Build history of the part. All positions in model axes, mm. Round coordinates to 2 decimals unless told otherwise and drop trailing zeros. Write each loop counter-clockwise with the first axis right and the second up, starting at its lowest first coordinate (ties: lowest second). Pieces come first, ordered by that corner, then holes. Notation, with made-up numbers: (14, 46) - (28, 46) arc R9 ccw to (28, 53) - close; hole circle Ø6 at (-9, 29.5). An arc over 180 degrees is marked (long way). Answer as a JSON object with one key per item and string values. Group by question number.
Item 1: Two-plate mould, pull along Z, no slides. Class faces 1 (the cylindrical face through (-31.156, 4.014, 32.365)), 2 (the flat face through (41, 33, 22)): +Z half, -Z half, draft (parallel to the pull), parting line (faces both ways), or undercut.
Item 2: Slice it at C-C, the plane y = 30. List the corners of the cut face in (x, z).
Item 3: Slice it at D-D, the plane x = 43.5. List the corners of the cut face in (y, z).
Item 4: Slice it at A-A, the plane z = 0. List the corners of the cut face in (x, y).
Item 5: Flat gauge pins, fed straight in: pin 1 (5 mm diameter, centred on x = 36, z = -23, fed in from +Y); pin 2 (2 mm diameter, centred on x = 20.5, y = 11.5, fed in from -Z); pin 3 (12 mm diameter, centred on y = 20.5, z = 27, fed in from -X). Where does each tip first touch, or does it go through?
Item 6: Probe line 1 (X direction, y = 2.3, z = 0); line 2 (Y direction, x = 3, z = 40); line 3 (Z direction, x = -8.5, y = 24). List the from-to ranges inside material, lowest first. Write a range as from..to.
Item 7: Slice it at B-B, the plane x = 0. List the corners of the cut face in (y, z), then the cut area to 3 significant figures.
from build123d import *

# Parameters (mm, degrees)
SKETCH1_R           = 50
BOSS_EXTRUDE1_DEPTH = 5
SKETCH2_R           = 2.5
BOSS_EXTRUDE2_DEPTH = 30
SKETCH3_R           = 50
BOSS_EXTRUDE3_DEPTH = 28
SKETCH4_R           = 39
CUT_EXTRUDE1_DEPTH  = 6
SKETCH5_R           = 3
CUT_EXTRUDE2_DEPTH  = 44
SKETCH6_R           = 50
SKETCH6_R_2         = 39
BOSS_EXTRUDE4_DEPTH = 3


with BuildPart() as part:
    # Sketch1 → Boss-Extrude1 (new body)
    with BuildSketch(Plane(origin=(0, 0, 0), x_dir=(1, 0, 0), z_dir=(0, 1, 0))):
        Circle(SKETCH1_R)
    extrude(amount=BOSS_EXTRUDE1_DEPTH)

    # Sketch2 → Boss-Extrude2 (add)
    with BuildSketch(Plane(origin=(0, 5, 0), x_dir=(1, 0, 0), z_dir=(0, 1, 0))):
        with Locations((43, 0)):
            Circle(SKETCH2_R)
        with Locations((36.173901912, -23.247555151)):
            Circle(SKETCH2_R)
        with Locations((17.862845559, -39.1141758)):
            Circle(SKETCH2_R)
        with Locations((-6.119538046, -42.562322001)):
            Circle(SKETCH2_R)
        with Locations((-28.15901156, -32.497231697)):
            Circle(SKETCH2_R)
        with Locations((-41.258197865, -12.114499944)):
            Circle(SKETCH2_R)
        with Locations((-41.258197865, 12.114499944)):
            Circle(SKETCH2_R)
        with Locations((-28.15901156, 32.497231697)):
            Circle(SKETCH2_R)
        with Locations((-6.119538046, 42.562322001)):
            Circle(SKETCH2_R)
        with Locations((17.862845559, 39.1141758)):
            Circle(SKETCH2_R)
        with Locations((36.173901912, 23.247555151)):
            Circle(SKETCH2_R)
    extrude(amount=BOSS_EXTRUDE2_DEPTH)

    # Sketch3 → Boss-Extrude3 (add)
    with BuildSketch(Plane(origin=(0, 5, 0), x_dir=(1, 0, 0), z_dir=(0, 1, 0))):
        Circle(SKETCH3_R)
        with BuildLine():
            ThreePointArc((45.918604651, -2.735278211), (47, 0), (45.918604651, 2.735278211))
            ThreePointArc((45.918604651, 2.735278211), (44.136676786, 12.959697615), (40.107991433, 22.524409497))
            ThreePointArc((40.107991433, 22.524409497), (39.538916043, 25.41011842), (37.150385338, 27.126534413))
            ThreePointArc((37.150385338, 27.126534413), (30.123593761, 34.76448042), (21.563374325, 40.632756339))
            ThreePointArc((21.563374325, 40.632756339), (19.524505611, 42.752703782), (16.587181171, 42.905307606))
            ThreePointArc((16.587181171, 42.905307606), (6.546482561, 45.531786327), (-3.827461772, 45.840490141))
            ThreePointArc((-3.827461772, 45.840490141), (-6.688797399, 46.521607768), (-9.242335817, 45.061948789))
            ThreePointArc((-9.242335817, 45.061948789), (-19.109090598, 41.843071786), (-28.0031058, 36.494192217))
            ThreePointArc((-28.0031058, 36.494192217), (-30.778454495, 35.520229995), (-32.137476487, 32.911739623))
            ThreePointArc((-32.137476487, 32.911739623), (-38.69766251, 24.869477603), (-43.287961597, 15.561246119))
            ThreePointArc((-43.287961597, 15.561246119), (-45.09616976, 13.241430172), (-44.829195445, 10.312285671))
            ThreePointArc((-44.829195445, 10.312285671), (-46, 0), (-44.829195445, -10.312285671))
            ThreePointArc((-44.829195445, -10.312285671), (-45.09616976, -13.241430172), (-43.287961597, -15.561246119))
            ThreePointArc((-43.287961597, -15.561246119), (-38.69766251, -24.869477603), (-32.137476487, -32.911739623))
            ThreePointArc((-32.137476487, -32.911739623), (-30.778454495, -35.520229995), (-28.0031058, -36.494192217))
            ThreePointArc((-28.0031058, -36.494192217), (-19.109090598, -41.843071786), (-9.242335817, -45.061948789))
            ThreePointArc((-9.242335817, -45.061948789), (-6.688797399, -46.521607768), (-3.827461772, -45.840490141))
            ThreePointArc((-3.827461772, -45.840490141), (6.546482561, -45.531786327), (16.587181171, -42.905307606))
            ThreePointArc((16.587181171, -42.905307606), (19.524505611, -42.752703782), (21.563374325, -40.632756339))
            ThreePointArc((21.563374325, -40.632756339), (30.123593761, -34.76448042), (37.150385338, -27.126534413))
            ThreePointArc((37.150385338, -27.126534413), (39.538916043, -25.41011842), (40.107991433, -22.524409497))
            ThreePointArc((40.107991433, -22.524409497), (44.136676786, -12.959697615), (45.918604651, -2.735278211))
        make_face(mode=Mode.SUBTRACT)
    extrude(amount=BOSS_EXTRUDE3_DEPTH)

    # Sketch4 → Cut-Extrude1 (cut)
    with BuildSketch(Plane(origin=(0, 5, 0), x_dir=(1, 0, 0), z_dir=(0, 1, 0))):
        Circle(SKETCH4_R)
    extrude(amount=-CUT_EXTRUDE1_DEPTH, mode=Mode.SUBTRACT)

    # Sketch5 → Cut-Extrude2 (cut, symmetric)
    with BuildSketch(Plane(origin=(0, 5, 0), x_dir=(1, 0, 0), z_dir=(0, 1, 0))):
        with Locations((43, 0)):
            Circle(SKETCH5_R)
        with Locations((36.173901912, -23.247555151)):
            Circle(SKETCH5_R)
        with Locations((17.862845559, -39.1141758)):
            Circle(SKETCH5_R)
        with Locations((-6.119538046, -42.562322001)):
            Circle(SKETCH5_R)
        with Locations((-28.15901156, -32.497231697)):
            Circle(SKETCH5_R)
        with Locations((-41.258197865, -12.114499944)):
            Circle(SKETCH5_R)
        with Locations((-41.258197865, 12.114499944)):
            Circle(SKETCH5_R)
        with Locations((-28.15901156, 32.497231697)):
            Circle(SKETCH5_R)
        with Locations((-6.119538046, 42.562322001)):
            Circle(SKETCH5_R)
        with Locations((17.862845559, 39.1141758)):
            Circle(SKETCH5_R)
        with Locations((36.173901912, 23.247555151)):
            Circle(SKETCH5_R)
    extrude(amount=CUT_EXTRUDE2_DEPTH, both=True, mode=Mode.SUBTRACT)

    # Sketch6 → Boss-Extrude4 (add)
    with BuildSketch(Plane.XZ):
        Circle(SKETCH6_R)
        Circle(SKETCH6_R_2, mode=Mode.SUBTRACT)
    extrude(amount=-BOSS_EXTRUDE4_DEPTH)


solid = part.part
Geometry says:
{
 "1": {"face 1": "undercut", "face 2": "draft"},
 "2": {"outline": "circle Ø100 at (0, 0); hole (-44.83, -10.31) arc R4 ccw to (-43.29, -15.56) arc R46 ccw to (-32.14, -32.91) arc R4 ccw to (-28, -36.49) arc R46 ccw to (-9.24, -45.06) arc R4 ccw to (-3.83, -45.84) arc R46 ccw to (16.59, -42.91) arc R4 ccw to (21.56, -40.63) arc R46 ccw to (37.15, -27.13) arc R4 ccw to (40.11, -22.52) arc R46 ccw to (45.92, -2.74) arc R4 ccw to (45.92, 2.74) arc R46 ccw to (40.11, 22.52) arc R4 ccw to (37.15, 27.13) arc R46 ccw to (21.56, 40.63) arc R4 ccw to (16.59, 42.91) arc R46 ccw to (-3.83, 45.84) arc R4 ccw to (-9.24, 45.06) arc R46 ccw to (-28, 36.49) arc R4 ccw to (-32.14, 32.91) arc R46 ccw to (-43.29, 15.56) arc R4 ccw to (-44.83, 10.31) arc R46 ccw to start"},
 "3": {"outline": "(0, -24.65) - (33, -24.65) - (33, -14.96) - (5, -14.96) - (5, -2.96) - (3, -2.96) - (3, 2.96) - (5, 2.96) - (5, 14.96) - (33, 14.96) - (33, 24.65) - (0, 24.65) - close"},
 "4": {"outline": "(-50, 0) - (-39, 0) - (-39, 5) - (-46, 5) - (-46, 33) - (-50, 33) - close; (39, 0) - (50, 0) - (50, 33) - (47, 33) - (47, 5) - (46, 5) - (46, 3) - (40, 3) - (40, 5) - (39, 5) - close"},
 "5": {"pin 1": "stops at y = 3", "pin 2": "stops at z = -46.04", "pin 3": "stops at x = -45.38"},
 "6": {"line 1": "x = -50..-39, 39..50", "line 2": "y = 0..5", "line 3": "z = -49.27..-45.78, 45.78..49.27"},
 "7": {"outline": "(0, -50) - (33, -50) - (33, -46) - (5, -46) - (5, -39) - (0, -39) - close; (0, 39) - (5, 39) - (5, 46) - (33, 46) - (33, 50) - (0, 50) - close", "area": "334 mm^2"}
}
